Geometry check sheet. Reference: the model listing, model coordinates, mm. A direction names the side the tool comes from. Coordinates: 2 decimals unless noted, no trailing zeros. Loops run counter-clockwise (first coordinate to the right, second up) from the corner with the lowest first, then second, coordinate; pieces in that order, holes last. Notation, with made-up numbers: (9.5, 88.5) - (67.5, 88.5) arc R10 cw to (67.5, 103.5) - close; hole circle Ø4 at (1, 52.5). An arc over 180 degrees is marked (long way). One line per item, written item: value.
Autodesk Inventor part; units mm, degrees
ref_plane "YZ Plane" through (0, 0, 0) normal (1, 0, 0) x (0, 1, 0)
sketch "Skizze1" plane through (0, 0, 0) normal (0, 1, 0) x (-1, 0, 0)
  circle A0 centre (0, 0) radius 30
  circle A1 centre (0, 0) radius 27
  dimension "d0" = 60
  dimension "d1" = 54
extrude "Extrusion1" add sketch "Skizze1" along normal mid plane 10
sketch "Skizze5" plane through (0, 0, 0) normal (0, 1, 0) x (-1, 0, 0)
  line L0 (12.75, -14.75) -> (-12.75, -14.75)
  line L1 (-12.75, -14.75) -> (-12.75, 14.75)
  line L2 (-12.75, 14.75) -> (12.75, 14.75)
  line L3 (12.75, 14.75) -> (12.75, -14.75)
  line L4 (49.4097, 0) -> (-52.5504, 0) construction
  line L5 (0, -53.7913) -> (0, 68.1535) construction
  line L6 (-16.75, -18.75) -> (16.75, -18.75)
  line L7 (16.75, -18.75) -> (16.75, 18.75)
  line L8 (16.75, 18.75) -> (-16.75, 18.75)
  line L9 (-16.75, 18.75) -> (-16.75, -18.75)
  point P0 (0, 0)
  dimension "d33" = 29.5
  dimension "d34" = 25.5
  dimension "d35" = 4
extrude "Extrusion5" add sketch "Skizze5" along normal mid plane 2.5 contours L0 L1 L2 L3 | L9 L8 L7 L6
ref_plane "Arbeitsebene1" through (0, 0, 0) normal (0, 1, 0) x (-1, 0, 0)
chamfer "Fase1" distance 1 angle 45 2 edges at (30, 5, 0) (30, -5, 0)
sketch "Skizze2" plane through (0, 0, 0) normal (0, 1, 0) x (-1, 0, 0)
  line L0 (0, 42.2301) -> (0, -36.7007) construction
  line L1 (32.6355, 0) -> (-32.6355, 0) construction
  line L2 (16.5, 34.419) -> (16.5, -40.3324) construction
  line L3 (-16.5, 35.4304) -> (-16.5, -34.8157) construction
  line L4 (23.5881, 16.5) -> (-32.0387, 16.5) construction
  line L5 (23.5881, -16.5) -> (-39.8541, -16.5) construction
  circle A0 centre (16.5, -16.5) radius 1.75
  circle A1 centre (16.5, 16.5) radius 1.75
  circle A2 centre (-16.5, 16.5) radius 1.75
  circle A3 centre (-16.5, -16.5) radius 1.75
  circle A4 centre (-16.5, 16.5) radius 3.6749
  circle A5 centre (-16.5, -16.5) radius 3.7161
  circle A6 centre (16.5, -16.5) radius 3.7
  circle A7 centre (16.5, 16.5) radius 3.6747
  point P0 (0, 0)
  dimension "d8" = 33
  dimension "d9" = 33
  dimension "d10" = 3.5
  dimension "d11" = 3.5
  dimension "d12" = 3.5
  dimension "d13" = 3.5
extrude "Extrusion2" add sketch "Skizze2" along normal mid plane 2.5
ref_plane "Arbeitsebene2" through (0, 0, -30.5) normal (0, 0, 1) x (1, 0, 0)
extrude "Extrusion6" cut sketch "Skizze2" against normal mid plane 3 contours A0 | A1 | A2 | A3
sketch "Skizze12" plane through (0, 5, 0) normal (0, 1, 0) x (1, 0, 0)
  circle A0 centre (0, 0) radius 27
  circle A1 centre (0, 0) radius 31.5802
extrude "Extrusion13" cut sketch "Skizze12" against normal blind 10
sketch "Skizze13" plane through (0, 1.25, 0) normal (0, 1, 0) x (1, 0, 0)
  line L0 (-13.5947, -18.75) -> (13.5944, -18.75)
  line L1 (-13.5947, -18.75) -> (13.5944, -18.75)
  line L2 (13.5944, -18.75) -> (13.5944, -14.75)
  line L3 (13.5944, -14.75) -> (-13.5947, -14.75)
  line L4 (-13.5947, -14.75) -> (-13.5947, -18.75)
  point P0 (0, 0)
  dimension "d58" = 4
extrude "Extrusion14" cut sketch "Skizze13" against normal blind 3
fillet "Rundung4" radius 2 2 edges at (13.5944, 0, 14.75) (-13.5947, 0, 14.75)
sketch "Skizze14" plane through (0, 1.25, 0) normal (0, 1, 0) x (1, 0, 0)
  line L0 (-13, -12.25) -> (13, -12.25)
  line L1 (13, -12.25) -> (13, 13.75)
  line L2 (13, 13.75) -> (-13, 13.75)
  line L3 (-13, 13.75) -> (-13, -12.25)
  line L4 (0, -43.7267) -> (0, 49.5069) construction
  line L5 (-24.7381, 0) -> (29.5694, 0) construction
  line L6 (13.5425, 18.75) -> (-13.5627, 18.75) construction
  line L7 (-13, -12.25) -> (-16.75, -12.25)
  line L8 (-16.75, 12.8084) -> (-16.75, -12.8338)
  line L9 (-16.75, -12.25) -> (-16.75, 12.815)
  line L10 (-16.75, 12.815) -> (-13.0013, 18.75)
  line L11 (13, -12.25) -> (16.75, -12.25)
  line L12 (16.75, -12.8336) -> (16.75, 12.7924)
  arc A0 (16.75, 12.7924) -> (19.551, 18.6215) centre (16.5, 16.5) ccw
  line L13 (16.75, -12.25) -> (16.75, 12.7924)
  line L14 (16.75, 12.7924) -> (13.0013, 18.75)
  line L15 (13.0013, 18.75) -> (-13.0013, 18.75)
  point P0 (0, 0)
  dimension "d62" = 26
  dimension "d63" = 26
  dimension "d64" = 5
extrude "Extrusion15" add sketch "Skizze14" along normal blind 5 contours L7 L8 L9 L10 L15 L14 L12 L11 L1 L2 L3
sketch "Skizze15" plane through (0, 6.25, 0) normal (0, 1, 0) x (1, 0, 0)
  line L0 (-13, 13.75) -> (-13, -12.25)
  line L1 (13, 13.75) -> (-13, 13.75)
  line L2 (-13, -12.25) -> (-12, -12.25)
  line L3 (-12, -12.25) -> (-12, 13.75)
  line L4 (-12, 13.75) -> (-13, 13.75)
  line L5 (-13, 13.75) -> (-13, -12.25)
  line L6 (13, -12.25) -> (16.75, -12.25)
  line L7 (13, -12.25) -> (12, -12.25)
  line L8 (12, -12.25) -> (12, 13.75)
  line L9 (12, 13.75) -> (13, 13.75)
  line L10 (13, 13.75) -> (13, -12.25)
  point P0 (0, 0)
  dimension "d67" = 1
  dimension "d68" = 1
extrude "Extrusion16" add sketch "Skizze15" against normal blind 3
properties part number "_3D-Druck"
(1) Material ranges on probe 1 along Z at (x, y) = (16.5, 0.2); probe 2 along X at (y, z) = (-0.15, -16.5); probe 3 along X at (y, z) = (3.5, -1.5), recorded low to high. Write a range as from..to.
Reply:
probe 1: -20.22..-18.25, -14.75..14.75, 18.25..20.17
probe 2: -20.2..-18.25, -14.75..14.75, 18.25..20.22
probe 3: -16.75..-12, 12..16.75
(2) Release check for a two-part mould opening along Z. For faces 1 (the face through (0, 0, 14.75)), 2 (the face through (-16.75, 2, 0)), 3 (the face through (-14.902, 3.715, -15.741)) record: pulls with the +Z half, pulls with the -Z half, needs draft (parallel to the pull), parting line crosses it, or undercut.
Reply:
face 1: pulls with the +Z half
face 2: undercut
face 3: pulls with the -Z half
(3) Access from +Z, -Z, +X, -X, +Y, -Y to the whole of each face (thin tool, end or side, straight path). Record for faces 4 (the face through (14, 4, 12.25)), 5 (the face through (12, 5, -1)), 6 (the face through (16.75, 3, 0)), 7 (the face through (18.3, 1.25, -17.3)).
Reply:
face 4: +Z, +X, -X, +Y
face 5: +Z, +Y
face 6: +X, +Y, -Y
face 7: -Z, +X, +Y
(4) Cross-section at D-D on y = 3.75. Record the cut outline in (x, z) (3 decimals), and give its area (3 significant figures).
Reply:
outline: (-16.75, -12.815) - (-13.001, -18.75) - (13.001, -18.75) - (16.75, -12.792) - (16.75, 12.25) - (12, 12.25) - (12, -13.75) - (-12, -13.75) - (-12, 12.25) - (-16.75, 12.25) - close
area: 392 mm2
(5) Go/stop test with flat-tipped pins: pin 1 Ø2 at (x, y) = (-1, 0) entering from +Z; pin 2 Ø3 at (x, z) = (16.5, 16.5) entering from +Y; pin 3 Ø2.5 at (x, y) = (15, 3.5) entering from +Z; pin 4 Ø4 at (x, z) = (-15.5, 14.5) entering from +Y. Record where each tip stops, or that it passes through.
Reply:
pin 1: z = 14.75
pin 2: through
pin 3: z = 12.25
pin 4: y = 1.25
(6) Cross-section at B-B on z = -1. Record the cut outline in (x, y).
Reply:
outline: (-16.75, -1.25) - (16.75, -1.25) - (16.75, 6.25) - (12, 6.25) - (12, 3.25) - (13, 3.25) - (13, 1.25) - (-13, 1.25) - (-13, 3.25) - (-12, 3.25) - (-12, 6.25) - (-16.75, 6.25) - close
(7) Cross-section at A-A on y = 0. Record the cut outline in (x, z).
Reply:
outline: (-19.47, -18.7) arc R27 ccw to (-18.7, -19.47) arc R3.7 ccw to (-13.56, -18.75) - (13.54, -18.75) arc R3.72 ccw to (18.62, -19.55) arc R27 ccw to (19.55, -18.62) arc R3.72 ccw to (16.75, -12.79) - (16.75, 12.83) arc R3.67 ccw to (19.29, 18.89) arc R27 ccw to (18.89, 19.29) arc R3.67 ccw to (13.59, 18.75) - (13.59, 16.75) arc R2 cw to (11.59, 14.75) - (-11.59, 14.75) arc R2 cw to (-13.59, 16.75) - (-13.59, 18.75) arc R3.67 ccw to (-18.89, 19.29) arc R27 ccw to (-19.29, 18.89) arc R3.67 ccw to (-16.75, 12.83) - (-16.75, -12.81) arc R3.7 ccw to start; hole circle Ø3.5 at (-16.5, -16.5); hole circle Ø3.5 at (-16.5, 16.5); hole circle Ø3.5 at (16.5, -16.5); hole circle Ø3.5 at (16.5, 16.5)
(8) Cross-section at C-C on x = -16. Record the cut outline in (y, z).
Reply:
outline: (-1.25, -20.17) - (1.25, -20.17) - (1.25, -18.18) - (-1.25, -18.18) - close; (-1.25, -14.82) - (1.25, -14.82) - (1.25, -14) - (6.25, -14) - (6.25, 12.25) - (1.25, 12.25) - (1.25, 14.82) - (-1.25, 14.82) - close; (-1.25, 18.18) - (1.25, 18.18) - (1.25, 20.14) - (-1.25, 20.14) - close
